Drawing for the job (mm, zero at the part's lowest x, y, z). A direction names the side the tool comes from. Round coordinates to 2 decimals unless told otherwise and drop trailing zeros. Write each loop counter-clockwise with the first axis right and the second up, starting at its lowest first coordinate (ties: lowest second). Pieces come first, ordered by that corner, then holes. Notation, with made-up numbers: (34, -20) - (52, -20) arc R8 cw to (52, -8) - close; hole circle Ø7 at (18.5, -23.5). An arc over 180 degrees is marked (long way). Answer in a Markdown table with one row per item.
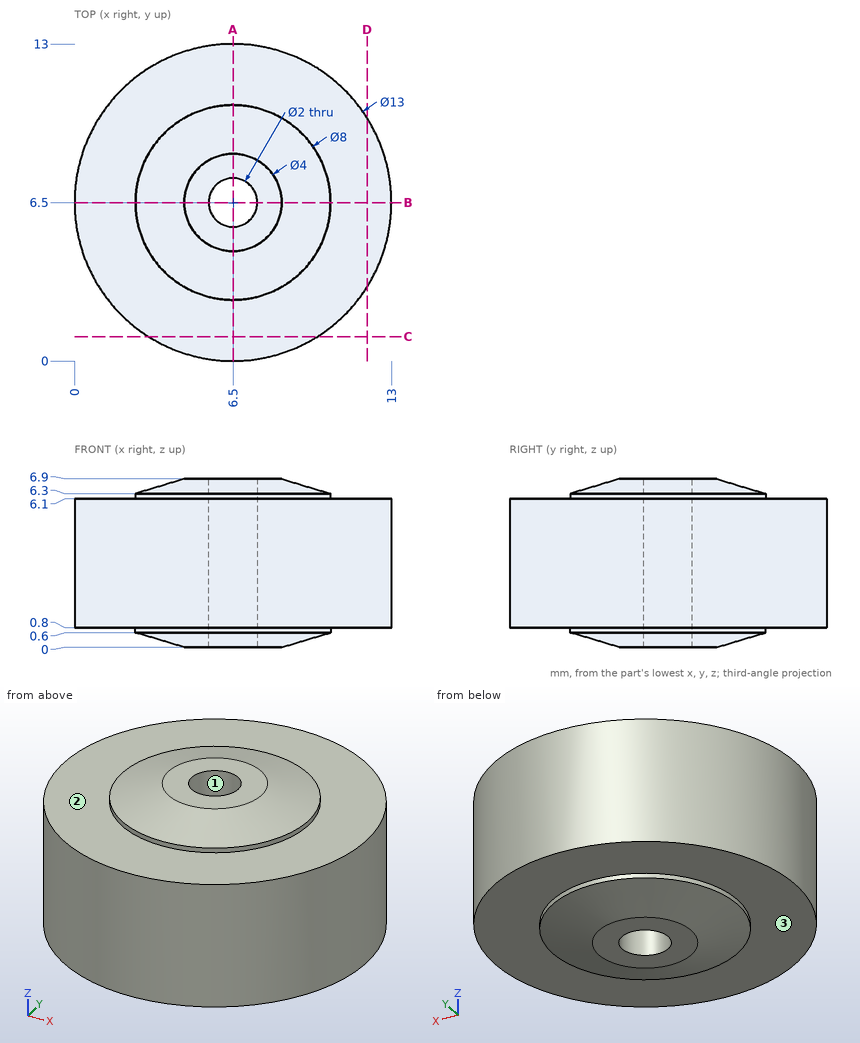
Q1. Drill centre lines: line 1 (Y direction, x = 6.5, z = 2.75); line 2 (Z direction, x = 2, y = 7.75); line 3 (Z direction, x = 3.25, y = 5.75). Where is each one in solid material? Low to high.
Computed:
| item | result |
|---|---|
| line 1 | y = 0 to 5.5, 7.5 to 13 |
| line 2 | z = 0.8 to 6.1 |
| line 3 | z = 0.4 to 6.5 |
Q2. 3-axis set-ups, long thin cutter, end or side, ignore diameter. For the marked faces 1, 2 and 3: which of +Z, -Z, +X, -X, +Y, -Y reach the whole face in a straight line?
Computed:
| item | result |
|---|---|
| face 1 | +Z, -Z |
| face 2 | +Z |
| face 3 | -Z |
Q3. Saw through at C-C on y = 1. List the corners of the cut face in (x, z), then the cut area to 3 significant figures.
Computed:
| item | result |
|---|---|
| outline | (3.04, 0.8) - (9.96, 0.8) - (9.96, 6.1) - (3.04, 6.1) - close |
| area | 36.7 mm2 |
Q4. Saw through at A-A on x = 6.5. List the corners of the cut face in (y, z).
Computed:
| item | result |
|---|---|
| outline | (0, 0.8) - (2.5, 0.8) - (2.5, 0.6) - (4.5, 0) - (5.5, 0) - (5.5, 6.9) - (4.5, 6.9) - (2.5, 6.3) - (2.5, 6.1) - (0, 6.1) - close; (7.5, 0) - (8.5, 0) - (10.5, 0.6) - (10.5, 0.8) - (13, 0.8) - (13, 6.1) - (10.5, 6.1) - (10.5, 6.3) - (8.5, 6.9) - (7.5, 6.9) - close |
Q5. Flat gauge pins, fed straight in: pin 1 (1.5 mm diameter, centred on x = 5.5, z = 1, fed in from +Y); pin 2 (1 mm diameter, centred on x = 4.5, z = 1, fed in from -Y); pin 3 (1.5 mm diameter, centred on x = 9.5, y = 8, fed in from +Z); pin 4 (1.8 mm diameter, centred on x = 6.5, y = 6.5, fed in from -Z). Where does each tip first touch, or does it go through?
Computed:
| item | result |
|---|---|
| pin 1 | stops at y = 13 |
| pin 2 | stops at y = 0.18 |
| pin 3 | stops at z = 6.72 |
| pin 4 | passes through |
